Answer from the drawing. Dimensions are ordinates in mm from the lowest x, y and z of the part. A direction names the side the tool comes from. Give positions to 0.01 mm unless a question says otherwise; leave off trailing zeros. Write each loop counter-clockwise with the first axis right and the second up, starting at its lowest first coordinate (ties: lowest second). Pieces come first, ordered by that corner, then holes.
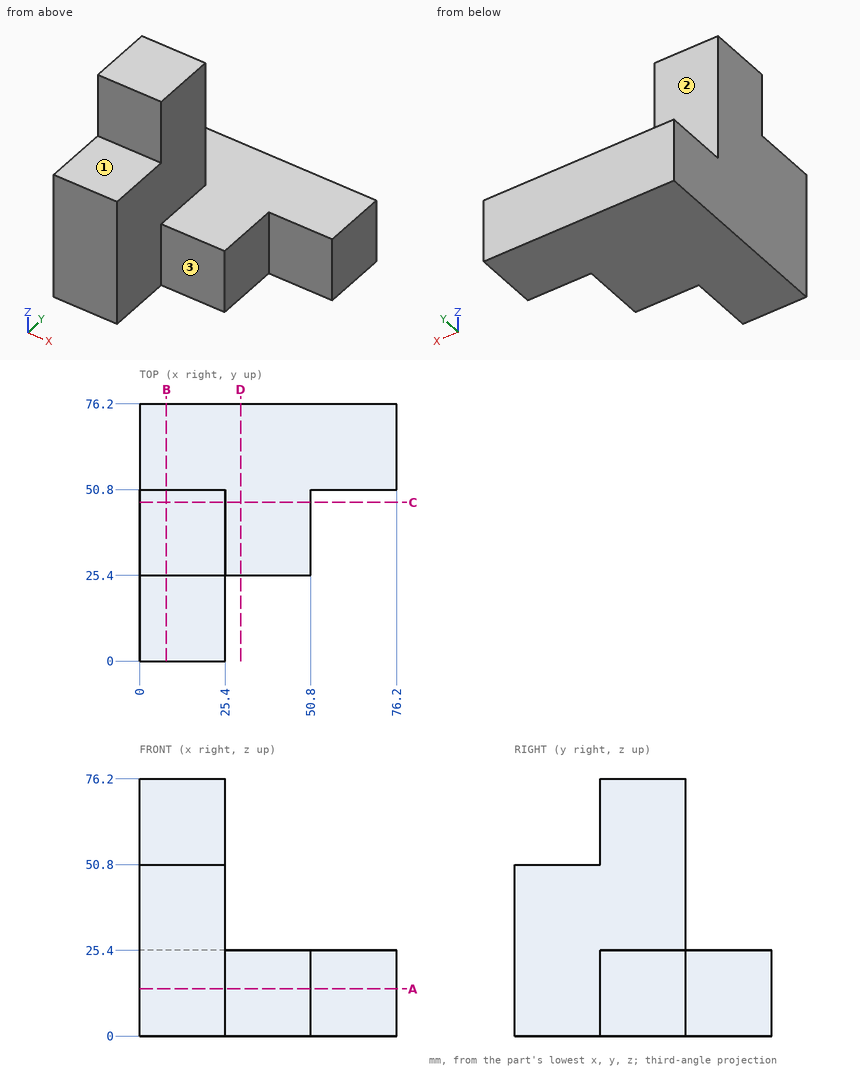
Item 1: Section B-B (x = 8) is taken. Write down the section's boundary in (y, z), and give its area (3 significant figures).
Result set:
outline: (0, 0) - (76.2, 0) - (76.2, 25.4) - (50.8, 25.4) - (50.8, 76.2) - (25.4, 76.2) - (25.4, 50.8) - (0, 50.8) - close
area: 3,870 mm2
Item 2: Section D-D (x = 30) is taken. Write down the section's boundary in (y, z).
Result set:
outline: (25.4, 0) - (76.2, 0) - (76.2, 25.4) - (25.4, 25.4) - close
Item 3: Which of the six approach directions +Z, -Z, +X, -X, +Y, -Y give full straight-line access (tool end or side, diameter ignored) to the marked faces 1, 2 and 3?
Result set:
face 1: +Z, +X, -X, -Y
face 2: +Z, +X, -X, +Y
face 3: +Z, -Z, +X, -Y
Item 4: Section A-A (z = 14) is taken. Write down the section's boundary in (x, y), and give its area (3 significant figures).
Result set:
outline: (0, 0) - (25.4, 0) - (25.4, 25.4) - (50.8, 25.4) - (50.8, 50.8) - (76.2, 50.8) - (76.2, 76.2) - (0, 76.2) - close
area: 3,870 mm2
Item 5: Each of these flat-tipped pins is pushed along its axis until it touches: pin 1 Ø1 at (x, y) = (14, 15) entering from +Z; pin 2 Ø1 at (x, z) = (10.5, 38) entering from +Y; pin 3 Ø6 at (x, y) = (68, 54.5) entering from +Z. Where does it stop, or does it pass through?
Result set:
pin 1: stops at z = 50.8
pin 2: stops at y = 50.8
pin 3: stops at z = 25.4
Item 6: Section C-C (y = 47) is taken. Write down the section's boundary in (x, z).
Result set:
outline: (0, 0) - (50.8, 0) - (50.8, 25.4) - (25.4, 25.4) - (25.4, 76.2) - (0, 76.2) - close
Item 7: Find the intervals of material crossed by line 1 along Z through (x, y) = (43, 69); line 2 along Y through (x, z) = (61, 17.5); line 3 along X through (y, z) = (32.5, 15.5), in increasing order.
Result set:
line 1: z = 0 to 25.4
line 2: y = 50.8 to 76.2
line 3: x = 0 to 50.8
